CAD build for the part. Positions are in the model's coordinates, mm. Face numbers are marked on the shaded views. A direction names the side the tool comes from. Round coordinates to 2 decimals unless told otherwise and drop trailing zeros. Write each loop counter-clockwise with the first axis right and the second up, starting at its lowest first coordinate (ties: lowest second). Pieces come first, ordered by that corner, then holes. Notation, with made-up numbers: M 82.5,8 L 89.5,8 A14 cw 89.5,15 Z; hole C 82.5,55.5 d5. An arc over 180 degrees is marked long. Write each question's results on one line, items separated by ' | '. Start each with the question number.
```python
from build123d import *

# Parameters (mm, degrees)
SKETCH1_R           = 2
BOSS_EXTRUDE1_DEPTH = 6
BOSS_EXTRUDE2_DEPTH = 25
CUT_EXTRUDE1_DEPTH  = 26


with BuildPart() as part:
    # Sketch1 → Boss-Extrude1 (new body)
    with BuildSketch(Plane.XY):
        Polygon((-12.416, -27.1625), (-37.5, -27.1625), (-37.5, 117.1625), (-12.666, 117.1625), (-12.666, 76.912960749), (27.667562569, 76.912960749), (29.262581996, 72.162960749), (-12.416, 72.162960749), align=None)
        with BuildLine():
            ThreePointArc((-37.5, -103.068178229), (-27.5324139, -102.499769625), (-37.5, -101.931361022))
            Line((-37.5, -101.931361022), (-37.5, -27.1625))
            Line((-37.5, -27.1625), (-12.416, -27.1625))
            Line((-12.416, -27.1625), (-12.416, -117.1625))
            Line((-12.416, -117.1625), (-37.5, -117.1625))
            Line((-37.5, -117.1625), (-37.5, -103.068178229))
        make_face()
        Polygon((-12.416, -117.1625), (37.5, -117.1625), (37.5, 47.631763907), (29.262581996, 72.162960749), (-12.416, 72.162960749), (-12.416, -27.1625), align=None)
        with Locations((-2.542, -102.503947692)):
            Circle(SKETCH1_R, mode=Mode.SUBTRACT)
        with Locations((32.5324139, -102.503947692)):
            Circle(SKETCH1_R, mode=Mode.SUBTRACT)
    extrude(amount=BOSS_EXTRUDE1_DEPTH)

    # Sketch1_4 → Boss-Extrude2 (add)
    with BuildSketch(Plane.XY):
        Polygon((-12.416, -27.1625), (-37.5, -27.1625), (-37.5, 117.1625), (-12.666, 117.1625), (-12.666, 76.912960749), (27.667562569, 76.912960749), (29.262581996, 72.162960749), (-12.416, 72.162960749), align=None)
        with BuildLine():
            ThreePointArc((-37.5, -103.068178229), (-27.5324139, -102.499769625), (-37.5, -101.931361022))
            Line((-37.5, -101.931361022), (-37.5, -27.1625))
            Line((-37.5, -27.1625), (-12.416, -27.1625))
            Line((-12.416, -27.1625), (-12.416, -117.1625))
            Line((-12.416, -117.1625), (-37.5, -117.1625))
            Line((-37.5, -117.1625), (-37.5, -103.068178229))
        make_face()
    extrude(amount=BOSS_EXTRUDE2_DEPTH)

    # Sketch2 → Cut-Extrude1 (cut)
    with BuildSketch(Plane(origin=(-12.416, 0, 0), x_dir=(0, 0, -1), z_dir=(1, 0, 0))):
        Polygon((-25, -27.1625), (-6, -117.1625), (-25, -117.1625), align=None)
    extrude(amount=-CUT_EXTRUDE1_DEPTH, mode=Mode.SUBTRACT)


solid = part.part
```
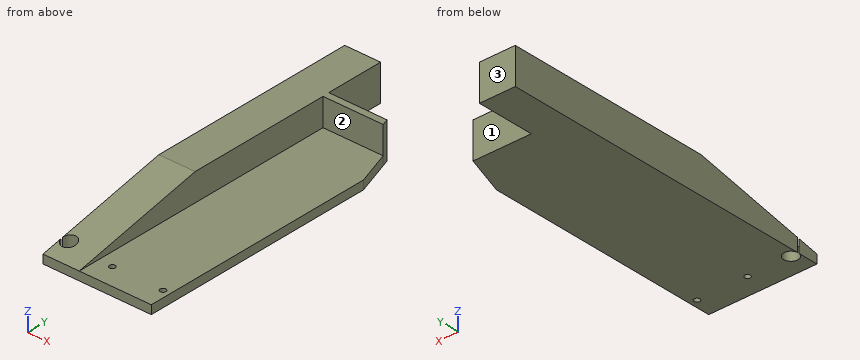
1) Wall check: line 1 along X through (y, z) = (3, 21); line 2 along Z through (x, y) = (28.5, 50); line 3 along Y through (x, z) = (8.5, 17). Give the ranges that are in metal, low to high. Write a range as from..to.
2) Saw through at B-B, the plane y = 28.5. Write the cut outline in (x, z).
3) Saw through at A-A, the plane x = 9. Write the cut outline in (y, z), plus the area to 3 significant figures.
4) Drop flat-ended pins along their axis: pin 1 Ø1.5 at (x, z) = (-1, 9) entering from +Y; pin 2 Ø1 at (x, y) = (-27.5, -83) entering from +Z; pin 3 Ø3 at (x, y) = (25, -2.5) entering from +Z; pin 4 Ø11.5 at (x, y) = (-32.53, -102.5) entering from -Z. Give the stop position or say it passes through.
5) Saw through at D-D, the plane x = -33. Write the cut outline in (y, z), plus the area to 3 significant figures.
6) 3-axis set-ups, long thin cutter, end or side, ignore diameter. For the marked faces 1, 2 and 3: which of +Z, -Z, +X, -X, +Y, -Y reach the whole face in a straight line?
7) Saw through at C-C, the plane z = 4. Write the cut outline in (x, y).
Filled sheet:
1) line 1: x = -37.5..-12.42 | line 2: z = 0..6 | line 3: y = 72.16..76.91
2) outline: M -37.5,0 L 37.5,0 L 37.5,6 L -12.42,6 L -12.42,25 L -37.5,25 Z
3) outline: M -117.16,0 L 76.91,0 L 76.91,25 L 72.16,25 L 72.16,6 L -117.16,6 Z | area: 1,250 mm^2
4) pin 1: stops at y = 76.91 | pin 2: stops at z = 13.32 | pin 3: stops at z = 6 | pin 4: stops at z = 0
5) outline: M -117.16,0 L -107.48,0 L -107.48,8.04 L -117.16,6 Z; M -97.52,0 L 117.16,0 L 117.16,25 L -27.16,25 L -97.52,10.15 Z | area: 4,910 mm^2
6) face 1: +Z, -Z, +X, +Y | face 2: +Z, +X, -Y | face 3: +Z, -Z, +X, -X, +Y
7) outline: M -37.5,-117.16 L 37.5,-117.16 L 37.5,47.63 L 27.67,76.91 L -12.67,76.91 L -12.67,117.16 L -37.5,117.16 L -37.5,-101.93 A5 cw long -37.5,-103.07 Z; hole C -2.54,-102.5 d4; hole C 32.53,-102.5 d4
